```python
from build123d import *

# Parameters (mm, degrees)
F0_W      = 76.2
F0_H      = 38.1
F1_DEPTH  = 3.175
F2_R      = 5.08
F3_W      = 63.5
F3_H      = 38.1
F4_DEPTH  = 25.4
F5_W      = 50.8
F5_H      = 19.05
F6_DEPTH  = 25.4
F7_R      = 12.7
F8_DEPTH  = 28.576
F9_W      = 11.075838387
F9_H      = 15.6388808947
F10_DEPTH = 25.4
F11_R     = 5.08
F12_W     = 11.7130865455
F12_H     = 15.6796150815
F13_DEPTH = 25.4
F14_R     = 5.08


with BuildPart() as f1:
    # F0 (on Top) → F1 (new body)
    with BuildSketch(Plane.XY):
        Rectangle(F0_W, F0_H)
    extrude(amount=F1_DEPTH)

    # F2
    f2_edges = [f1.edges().sort_by_distance(p)[0] for p in [
        (-38.1, 19.05, 1.5875),
        (38.1, 19.05, 1.5875),
    ]]
    fillet(f2_edges, radius=F2_R)

    # F3 (on face) → F4 (join)
    with BuildSketch(Plane.XY.offset(3.175)):
        Rectangle(F3_W, F3_H)
    extrude(amount=F4_DEPTH)

    # F5 (on face) → F6 (cut)
    with BuildSketch(Plane.XY.offset(28.575)):
        with Locations((0, -9.525)):
            Rectangle(F5_W, F5_H)
    extrude(amount=-F6_DEPTH, mode=Mode.SUBTRACT)

    # F7 (on face) → F8 (cut, through all)
    with BuildSketch(Plane.XY.offset(28.575)):
        with Locations((0, 19.05)):
            Circle(F7_R)
    extrude(amount=-F8_DEPTH, mode=Mode.SUBTRACT)

    # F9 (on face) → F10 (cut)
    with BuildSketch(Plane.XY.offset(28.575)):
        with Locations((-26.2120808065, 11.2305595526)):
            Rectangle(F9_W, F9_H)
    extrude(amount=-F10_DEPTH, mode=Mode.SUBTRACT)

    # F11
    f11_edges = [f1.edges().sort_by_distance(p)[0] for p in [
        (-20.674162, 3.411119, 15.875),
    ]]
    fillet(f11_edges, radius=F11_R)

    # F12 (on face) → F13 (cut)
    with BuildSketch(Plane.XY.offset(28.575)):
        with Locations((25.8934567273, 11.2101924593)):
            Rectangle(F12_W, F12_H)
    extrude(amount=-F13_DEPTH, mode=Mode.SUBTRACT)

    # F14
    f14_edges = [f1.edges().sort_by_distance(p)[0] for p in [
        (20.036913, 3.370385, 15.875),
    ]]
    fillet(f14_edges, radius=F14_R)


solid = f1.part
```
Check sheet for the modelled part. Datum: model origin and axes. Units: mm. A direction names the side the tool comes from. Give positions to 0.01 mm unless a question says otherwise; leave off trailing zeros. Order: outer loops, then holes, each group sorted by start corner. A loop starts at its lowest first (then second) coordinate and runs counter-clockwise, first axis right, second up. Notation, with made-up numbers: (25.25, -39) -> (73.25, -39) arc R23 cw to (73.25, -4) -> close; hole circle Ø7 at (-2.75, 31). An arc over 180 degrees is marked (long way). Return JSON: item names as keys, results as strings.
1. Cross-section at A-A, the plane z = 4.5. Record the cut outline in (x, y).
From the geometry:
{"outline": "(-31.75, -19.05) -> (-25.4, -19.05) -> (-25.4, 0) -> (25.4, 0) -> (25.4, -19.05) -> (31.75, -19.05) -> (31.75, 3.37) -> (25.12, 3.37) arc R5.08 cw to (20.04, 8.45) -> (20.04, 19.05) -> (12.7, 19.05) arc R12.7 cw to (-12.7, 19.05) -> (-20.67, 19.05) -> (-20.67, 8.49) arc R5.08 cw to (-25.75, 3.41) -> (-31.75, 3.41) -> close"}
2. Mould release check, pull along X, two halves, no side actions. Record for faces 1 (the flat face through (-20.674, 14, 16)), 2 (the flat face through (-25.4, -10, 16)), 3 (the cylindrical face through (36.651, 17.522, 1.61)): +X half, -X half, draft (parallel to the pull), parting line (faces both ways), or undercut.
From the geometry:
{"face 1": "-X half", "face 2": "undercut", "face 3": "+X half"}
3. Cross-section at C-C, the plane x = 0. Record the cut outline in (y, z) (3 decimals).
From the geometry:
{"outline": "(-19.05, 0) -> (6.35, 0) -> (6.35, 28.575) -> (0, 28.575) -> (0, 3.175) -> (-19.05, 3.175) -> close"}
4. Material ranges on probe 1 along X at (y, z) = (-4, 22.5); probe 2 along Z at (x, y) = (-28, 15.5) (3 decimals); probe 3 along Y at (x, z) = (31, 9), recorded low to high. Write a range as [from, to].
From the geometry:
{"probe 1": "[-31.75, -25.4], [25.4, 31.75]", "probe 2": "[0, 3.175]", "probe 3": "[-19.05, 3.37]"}
5. Cross-section at B-B, the plane y = -8.5. Record the cut outline in (x, z) (3 decimals).
From the geometry:
{"outline": "(-38.1, 0) -> (38.1, 0) -> (38.1, 3.175) -> (31.75, 3.175) -> (31.75, 28.575) -> (25.4, 28.575) -> (25.4, 3.175) -> (-25.4, 3.175) -> (-25.4, 28.575) -> (-31.75, 28.575) -> (-31.75, 3.175) -> (-38.1, 3.175) -> close"}
6. Go/stop test with flat-tipped pins: P1, Ø9.5, axis at y = -9.5, z = 13, coming from the +X side; P2, Ø5.5, axis at y = -13, z = 14, coming from the -X side; P3, Ø3, axis at x = -18.5, z = 21.5, coming from the -Y side. Record where each tip stops, or that it passes through.
From the geometry:
{"P1": "x = 31.75", "P2": "x = -31.75", "P3": "y = 0"}
7. Cross-section at D-D, the plane y = 11. Record the cut outline in (x, z) (3 decimals), plus the area to 3 significant figures.
From the geometry:
{"outline": "(-38.1, 0) -> (-9.823, 0) -> (-9.823, 28.575) -> (-20.674, 28.575) -> (-20.674, 3.175) -> (-38.1, 3.175) -> close; (9.823, 0) -> (38.1, 0) -> (38.1, 3.175) -> (20.037, 3.175) -> (20.037, 28.575) -> (9.823, 28.575) -> close", "area": "715 mm^2"}
8. Set-up check for faces 4 (the flat face through (-29, 3.411, 16)), 5 (the flat face through (-31.75, -8, 16)), 6 (the flat face through (0, 0, 16)), 7 (the flat face through (28, 3.37, 16)), 8 (the flat face through (31.75, -8, 16)): record each of +Z, -Z, +X, -X, +Y, -Y from which the full face is reachable in a straight line by a thin tool's end or side.
From the geometry:
{"face 4": "+Z, -X, +Y", "face 5": "+Z, -X, +Y, -Y", "face 6": "+Z, -Y", "face 7": "+Z, +X, +Y", "face 8": "+Z, +X, +Y, -Y"}
